Input: part model. Units: mm. Frame: model coordinates. Face numbers are marked on the shaded views. A direction names the side the tool comes from. Round coordinates to 2 decimals unless told otherwise and drop trailing zeros. Write each loop counter-clockwise with the first axis right and the second up, starting at its lowest first coordinate (ties: lowest second). Pieces come first, ordered by that corner, then holes. Notation, with made-up numbers: (-16, -35) - (27, -35) arc R25 ccw to (27, 0) - close; hole circle Ø10 at (-0.5, -29). An arc over 180 degrees is marked (long way). Use one line per item in the form item = value.
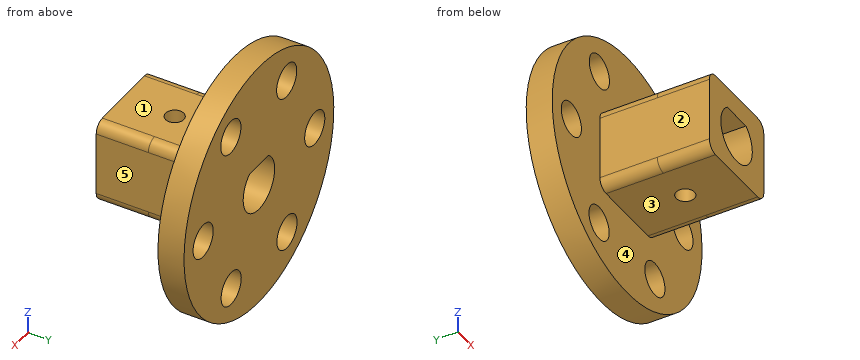
```python
from build123d import *

# Parameters (mm, degrees)
SKETCH_1_W                      = 30
SKETCH_1_H                      = 30
SKETCH_1_W_2                    = 21.5
SKETCH_1_H_2                    = 21.5
EXTRUDE_1_DEPTH                 = 5
SKETCH_2_W                      = 30
SKETCH_2_H                      = 30
EXTRUDE_2_DEPTH                 = 5
SKETCH_4_W                      = 17.554664
SKETCH_4_H                      = 16.21575
EXTRUDE_3_DEPTH                 = 11
SKETCH_5_R                      = 24.152219
SKETCH_5_R_2                    = 3.25
EXTRUDE_4_DEPTH                 = 5
CUT_EXTRUDE_2_DEPTH             = 21
FILLET_1_R                      = 2
SKETCH_10_W                     = 21.5
SKETCH_10_H                     = 21.5
EXTRUDE_5_DEPTH                 = 5
CUT_EXTRUDE_3_REACH             = 49.959
SKETCH_11_R                     = 1.75
CUT_EXTRUDE_3_DIRECTION_2_REACH = 49.959
SKETCH_12_R                     = 24.152219
CUT_EXTRUDE_4_DEPTH             = 21
CUT_EXTRUDE_5_REACH             = 42.096


with BuildPart() as part:
    # 草图1 → 凸台-拉伸1 (new body)
    with BuildSketch(Plane(origin=(0, 0, 0), x_dir=(1, 0, 0), z_dir=(0, 1, 0))):
        Rectangle(SKETCH_1_W, SKETCH_1_H)
        Rectangle(SKETCH_1_W_2, SKETCH_1_H_2, mode=Mode.SUBTRACT)
    extrude(amount=EXTRUDE_1_DEPTH)

    # 草图2 → 凸台-拉伸2 (add)
    with BuildSketch(Plane(origin=(0, 5, 0), x_dir=(1, 0, 0), z_dir=(0, 1, 0))):
        Rectangle(SKETCH_2_W, SKETCH_2_H)
    extrude(amount=EXTRUDE_2_DEPTH)

    # 草图4 → 凸台-拉伸3 (add)
    with BuildSketch(Plane(origin=(0, 10, 0), x_dir=(1, 0, 0), z_dir=(0, 1, 0))):
        Rectangle(SKETCH_4_W, SKETCH_4_H)
    extrude(amount=EXTRUDE_3_DEPTH)

    # 草图5 → 凸台-拉伸4 (add)
    with BuildSketch(Plane(origin=(0, 21, 0), x_dir=(1, 0, 0), z_dir=(0, 1, 0))):
        with Locations(Location((0, 0, 0), (0, 0, 270))):
            Circle(SKETCH_5_R)
        with Locations(Location((8.9491, 15.617734, 0), (0, 0, 270))):
            Circle(SKETCH_5_R_2, mode=Mode.SUBTRACT)
        with Locations(Location((17.999904, 0.058719, 0), (0, 0, 270))):
            Circle(SKETCH_5_R_2, mode=Mode.SUBTRACT)
        with Locations(Location((9.050804, -15.559015, 0), (0, 0, 270))):
            Circle(SKETCH_5_R_2, mode=Mode.SUBTRACT)
        with Locations(Location((-8.9491, -15.617734, 0), (0, 0, 270))):
            Circle(SKETCH_5_R_2, mode=Mode.SUBTRACT)
        with Locations(Location((-17.999904, -0.058719, 0), (0, 0, 270))):
            Circle(SKETCH_5_R_2, mode=Mode.SUBTRACT)
        with Locations(Location((-9.050804, 15.559015, 0), (0, 0, 270))):
            Circle(SKETCH_5_R_2, mode=Mode.SUBTRACT)
    extrude(amount=EXTRUDE_4_DEPTH)

    # 草图6 → 切除-拉伸2 (cut)
    with BuildSketch(Plane.XZ.offset(-5)):
        with BuildLine():
            Line((-3.024897, 4.075), (3.024897, 4.075))
            ThreePointArc((3.024897, 4.075), (0, -5.075), (-3.024897, 4.075))
        make_face()
    extrude(amount=-CUT_EXTRUDE_2_DEPTH, mode=Mode.SUBTRACT)

    # 圆角1
    fillet_1_edges = [part.edges().sort_by_distance(p)[0] for p in [
        (-8.777332, 15.5, -8.107875),
        (-8.777332, 15.5, 8.107875),
        (8.777332, 15.5, 8.107875),
        (8.777332, 15.5, -8.107875),
        (15, 5, 15),
        (-15, 5, 15),
        (-15, 5, -15),
        (15, 5, -15),
    ]]
    fillet(fillet_1_edges, radius=FILLET_1_R)

    # 草图10 → 凸台-拉伸5 (add)
    with BuildSketch(Plane.XZ.offset(-5)):
        Rectangle(SKETCH_10_W, SKETCH_10_H)
    extrude(amount=EXTRUDE_5_DEPTH)

    # 切除-拉伸3: up to this face of the body (flat: up to its plane)
    cut_extrude_3_end = Plane(part.part.faces().sort_by_distance((0, 5, -15))[0])
    # 草图11 → 切除-拉伸3 (cut, up to the picked face)
    with BuildSketch(Plane.XY.offset(8.107875), mode=Mode.PRIVATE) as cut_extrude_3_sk1:
        with Locations(Location((0.277648, 10, 0), (0, 0, 180))):
            Circle(SKETCH_11_R)
    cut_extrude_3_tool1 = split(extrude(cut_extrude_3_sk1.sketch, amount=-CUT_EXTRUDE_3_REACH, mode=Mode.PRIVATE), bisect_by=cut_extrude_3_end, keep=Keep.BOTH, mode=Mode.PRIVATE)
    add(cut_extrude_3_tool1.solids().sort_by(Axis((0.277648, 10, 8.107875), (0, 0, -1)))[0], mode=Mode.SUBTRACT)

    # 草图11 → 切除-拉伸3 direction 2 (cut, up to next)
    with BuildSketch(Plane.XY.offset(8.107875), mode=Mode.PRIVATE) as cut_extrude_3_direction_2_sk1:
        with Locations(Location((0.277648, 10, 0), (0, 0, 180))):
            Circle(SKETCH_11_R)
    cut_extrude_3_direction_2_tool1 = extrude(cut_extrude_3_direction_2_sk1.sketch, amount=CUT_EXTRUDE_3_DIRECTION_2_REACH, mode=Mode.PRIVATE) & part.part
    add(cut_extrude_3_direction_2_tool1.solids().sort_by_distance((0.277648, 10, 8.107875))[0], mode=Mode.SUBTRACT)

    # 草图12 → 切除-拉伸4 (cut)
    with BuildSketch(Plane.XZ.offset(-21)):
        with Locations(Location((0, 0, 0), (0, 0, 90))):
            Circle(SKETCH_12_R)
        with BuildLine():
            Line((-8.777332, -6.107875), (-8.777332, 6.107875))
            ThreePointArc((-8.777332, 6.107875), (-8.191546, 7.522088), (-6.777332, 8.107875))
            Line((-6.777332, 8.107875), (6.777332, 8.107875))
            ThreePointArc((6.777332, 8.107875), (8.191546, 7.522088), (8.777332, 6.107875))
            Line((8.777332, 6.107875), (8.777332, -6.107875))
            ThreePointArc((8.777332, -6.107875), (8.191546, -7.522088), (6.777332, -8.107875))
            Line((6.777332, -8.107875), (-6.777332, -8.107875))
            ThreePointArc((-6.777332, -8.107875), (-8.191546, -7.522088), (-8.777332, -6.107875))
        make_face(mode=Mode.SUBTRACT)
    extrude(amount=CUT_EXTRUDE_4_DEPTH, mode=Mode.SUBTRACT)

    # 草图13 → 切除-拉伸5 (cut, up to next)
    with BuildSketch(Plane(origin=(0, 5, 0), x_dir=(1, 0, 0), z_dir=(0, 1, 0)), mode=Mode.PRIVATE) as cut_extrude_5_sk1:
        with BuildLine():
            Line((-3.024897, -4.075), (3.024897, -4.075))
            ThreePointArc((3.024897, -4.075), (0, 5.075), (-3.024897, -4.075))
        make_face()
    cut_extrude_5_tool1 = extrude(cut_extrude_5_sk1.sketch, amount=-CUT_EXTRUDE_5_REACH, mode=Mode.PRIVATE) & part.part
    add(cut_extrude_5_tool1.solids().sort_by_distance((0, 5, -0.240279))[0], mode=Mode.SUBTRACT)


solid = part.part
```
(1) Cut plane D-D on x = 0. Output: boundary loops of the cut face in (y, z) (3 decimals).
Derived:
outline = (0, -8.108) - (8.272, -8.108) - (8.272, -5.075) - (0, -5.075) - close; (0, 4.075) - (8.272, 4.075) - (8.272, 8.108) - (0, 8.108) - close; (11.728, -8.108) - (21, -8.108) - (21, -24.152) - (26, -24.152) - (26, -5.075) - (11.728, -5.075) - close; (11.728, 4.075) - (26, 4.075) - (26, 24.152) - (21, 24.152) - (21, 8.108) - (11.728, 8.108) - close
(2) Cut plane C-C on z = -4. Output: boundary loops of the cut face in (x, y).
Derived:
outline = (-23.82, 21) - (-8.78, 21) - (-8.78, 0) - (-3.12, 0) - (-3.12, 26) - (-23.82, 26) - close; (3.12, 0) - (8.78, 0) - (8.78, 21) - (23.82, 21) - (23.82, 26) - (3.12, 26) - close
(3) Cut plane B-B on x = 16. Output: boundary loops of the cut face in (y, z), then the cut area to 3 significant figures.
Derived:
outline = (21, -18.09) - (26, -18.09) - (26, -2.62) - (21, -2.62) - close; (21, 2.5) - (26, 2.5) - (26, 18.09) - (21, 18.09) - close
area = 155 mm^2
(4) First-contact query: pin 1 Ø4.5 at (x, y) = (0.28, 10) entering from +Z; pin 2 Ø7.5 at (x, z) = (8.95, -15.62) entering from -Y; pin 3 Ø12 at (x, y) = (1.5, 8.5) entering from -Z; pin 4 Ø4 at (x, z) = (-8.95, 15.62) entering from +Y. Flat tips, straight axial feed; report the tip coordinate or a pass-through.
Derived:
pin_1 = 8.11
pin_2 = 21
pin_3 = -8.11
pin_4 = through
(5) Access query for the marked faces 1, 2, 3, 4 and 5. Directions: +Z, -Z, +X, -X, +Y, -Y. A direction counts if a zero-diameter tool reaches every point of the face in a straight line with its end or side. Return the directions, or none.
Derived:
face_1 = +Z, +X, -X, -Y
face_2 = +Z, -Z, -X, -Y
face_3 = -Z, +X, -X, -Y
face_4 = -Y
face_5 = +Z, -Z, +X, -Y
(6) Cut plane A-A on y = 15. Output: boundary loops of the cut face in (x, z) (3 decimals), then the cut area to 3 significant figures.
Derived:
outline = (-8.777, -6.108) arc R2 ccw to (-6.777, -8.108) - (6.777, -8.108) arc R2 ccw to (8.777, -6.108) - (8.777, 6.108) arc R2 ccw to (6.777, 8.108) - (-6.777, 8.108) arc R2 ccw to (-8.777, 6.108) - close; hole (-3.025, 4.075) arc R5.075 ccw (long way) to (3.025, 4.075) - close
area = 204 mm^2
(7) Material intervals for L1, parallel to X at y = 23.75, z = -17; L2, parallel to Y at x = 10, z = 7; L3, parallel to X at y = 22, z = 15, sorted ascending.
Derived:
L1 = -17.16 to -11.96, -6.14 to 6.01, 11.89 to 17.16
L2 = 21 to 26
L3 = -18.93 to -12.14, -5.76 to 5.85, 12.25 to 18.93
